Autodesk Inventor part; units mm, degrees
ref_plane "YZ Plane" through (0, 0, 0) normal (1, 0, 0) x (0, 1, 0)
ref_plane "XZ Plane" through (0, 0, 0) normal (0, 1, 0) x (-1, 0, 0)
ref_plane "XY Plane" through (0, 0, 0) normal (0, 0, 1) x (1, 0, 0)
sketch "Base" plane through (0, 0, 0) normal (0, 0, 1) x (1, 0, 0)
  circle A0 centre (0, 0) radius 34.1376
  circle A1 centre (0, 23.8125) radius 1.9939
  circle A2 centre (20.6222, 11.9063) radius 1.9939
  circle A3 centre (20.6222, -11.9062) radius 1.9939
  circle A4 centre (0, -23.8125) radius 1.9939
  circle A5 centre (-20.6222, -11.9062) radius 1.9939
  circle A6 centre (-20.6222, 11.9063) radius 1.9939
  circle A7 centre (0, 0) radius 12.25
  dimension "d2" = 68.2752
  dimension "d9" = 24.5
extrude "BaseFeature" add sketch "Base" along normal blind 4
equation "\"BendRadius\" = Thickness"
equation "\"BendReliefWidth\" = Thickness"
equation "\"BendReliefDepth\" = 0.5 * Thickness"
equation "\"CornerReliefSize\" = 4 * Thickness"
equation "\"MinimumRemnant\" = 2 * Thickness"
equation "\"TransitionRadius\" = BendRadius"
equation "\"JacobiRadiusSize\" = BendRadius"
equation "\"GapSize\" = Thickness"
equation "\"d6\" = Thickness"
properties part number "WheelSproketHub"
Read the model definition and answer for the solid it produces. Units are mm, in the model's axes. Round coordinates to 2 decimals unless told otherwise and drop trailing zeros. Order: outer loops, then holes, each group sorted by start corner. A loop starts at its lowest first (then second) coordinate and runs counter-clockwise, first axis right, second up.
1) The part is cut by section C-C on z = 3. Write down the section's boundary in (x, y).
2) The part is cut by section D-D on x = 21. Write down the section's boundary in (y, z), plus the area to 3 significant figures.
3) The part is cut by section A-A on y = 0. Write down the section's boundary in (x, z), plus the area to 3 significant figures.
4) The mould has two halves that part along Y. Classify faces 1 (the face through (0, -15, 0)), 2 (the face through (6.586, -10.329, 1.972)), 3 (the face through (-7.4, 33.326, 1.972)): released by +Y, released by -Y, zero draft, split by the parting line, or undercut.
5) Straight lines are drawn through the part: L1, parallel to Y at x = 0, z = 3.15; L2, parallel to Y at x = 20, z = 3.7; L3, parallel to X at y = -13, z = 2.45. For each, find the intervals that lie inside material, in ascending order.
6) The part is cut by section B-B on x = 0. Write down the section's boundary in (y, z), plus the area to 3 significant figures.
7) Flat-ended cylindrical pins translate along their axes: pin 1 (22 mm diameter, centred on x = 0, y = 0, fed in from +Z); pin 2 (1 mm diameter, centred on y = -16.5, z = 1, fed in from +X). Find the tip coordinate at first contact, or state that the pin passes through.
Resolved:
1. outline: circle Ø68.28 at (0, 0); hole circle Ø3.99 at (-20.62, -11.91); hole circle Ø3.99 at (-20.62, 11.91); hole circle Ø24.5 at (0, 0); hole circle Ø3.99 at (0, -23.81); hole circle Ø3.99 at (0, 23.81); hole circle Ø3.99 at (20.62, -11.91); hole circle Ø3.99 at (20.62, 11.91)
2. outline: (-26.91, 0) - (-13.86, 0) - (-13.86, 4) - (-26.91, 4) - close; (-9.95, 0) - (9.95, 0) - (9.95, 4) - (-9.95, 4) - close; (13.86, 0) - (26.91, 0) - (26.91, 4) - (13.86, 4) - close
2. area: 184 mm2
3. outline: (-34.14, 0) - (-12.25, 0) - (-12.25, 4) - (-34.14, 4) - close; (12.25, 0) - (34.14, 0) - (34.14, 4) - (12.25, 4) - close
3. area: 175 mm2
4. face 1: zero draft
4. face 2: undercut
4. face 3: split by the parting line
5. L1: y = -34.14 to -25.81, -21.82 to -12.25, 12.25 to 21.82, 25.81 to 34.14
5. L2: y = -27.67 to -13.8, -10.01 to 10.01, 13.8 to 27.67
5. L3: x = -31.57 to -22.29, -18.96 to 18.96, 22.29 to 31.57
6. outline: (-34.14, 0) - (-25.81, 0) - (-25.81, 4) - (-34.14, 4) - close; (-21.82, 0) - (-12.25, 0) - (-12.25, 4) - (-21.82, 4) - close; (12.25, 0) - (21.82, 0) - (21.82, 4) - (12.25, 4) - close; (25.81, 0) - (34.14, 0) - (34.14, 4) - (25.81, 4) - close
6. area: 143 mm2
7. pin 1: passes through
7. pin 2: stops at x = 30.16
